Geometry: final body of the model. Coordinates: model frame, mm. Coordinates: 2 decimals unless noted, no trailing zeros. Answer in a Markdown table with one row per item. Add a question column.
1) Ray query, line 1 (X direction, y = 6.5, z = 12.1); line 2 (X direction, y = 5.9, z = 6.5); line 3 (Y direction, x = 6.5, z = 6.9). Return the intervals inside material, ascending. Write a range as from..to.
2) Contact query for flat-ended pins moving along their axis: P1, Ø3.5, axis at x = 7.5, z = 5, coming from the -Y side; P2, Ø5.5, axis at x = 6.5, y = 19.5, coming from the +Z side; P3, Ø5, axis at x = 6.5, z = 6.5, coming from the -Y side. Output: stop coordinate, or through.
3) Section query A-A on z = 8. Count the separate pieces of the cut face and the enclosed holes in it, then the cut area to 3 significant figures.
Solid Edge part; units mm, degrees
sketch "Sketch1" plane through (0, 0, 0) normal (0, 0, 1) x (1, 0, 0)
  line L0 (39, 0) -> (39, 26)
  line L1 (39, 26) -> (0, 26)
  line L2 (0, 26) -> (0, 0)
  line L3 (0, 0) -> (39, 0)
extrude "Protrusion1" add sketch "Sketch1" along normal blind 13
sketch "Sketch2" plane through (6.5, 32.5, 6.5) normal (-1, 0, 0) x (0, -1, 0)
  line L0 (29, 6.5) -> (26, 6.5)
  line L1 (26, 6.5) -> (26, 0)
  line L2 (29, 0) -> (26, 0)
  line L3 (29, 0) -> (29, 1)
  line L4 (29, 1) -> (29.3967, 3.25)
  line L5 (29, 5.5) -> (29.3967, 3.25)
  line L6 (29, 6.5) -> (29, 5.5)
revolve "RevolvedCutout1" cut sketch "Sketch2" angle 360 about axis through (6.5, 6.5, 13) along (0, 0, -1)
chamfer "Chaflán_1" distance 0.75 angle 45 1 edges at (3.5, 6.5, 13)
pattern_linear "Pattern1" count 2 spacing 13 along (0, 1, 0) count 3 spacing 13 along (1, 0, 0) of "RevolvedCutout1", "Chaflán_1"
sketch "Sketch3" plane through (6.5, 32.5, 6.5) normal (-1, 0, 0) x (0, -1, 0)
  line L0 (31.5, 3) -> (32.5, 3)
  line L1 (32.5, 3) -> (32.5, 0)
  line L2 (32.5, 0) -> (31.5, 0)
  line L3 (31.5, 0) -> (26, 0)
  line L4 (26, 0) -> (26, 3)
  line L5 (26, 3) -> (27, 3)
  line L6 (27, 3) -> (29.25, 3.3967)
  line L7 (31.5, 3) -> (29.25, 3.3967)
revolve "RevolvedCutout2" cut sketch "Sketch3" angle 360 about axis through (6.5, 1, 6.5) along (0, 1, 0)
chamfer "Chaflán_2" distance 0.75 angle 45 1 edges at (6.5, 0, 3.5)
pattern_linear "Pattern3" count 3 spacing 13 along (1, 0, 0) of "RevolvedCutout2", "Chaflán_2"
chamfer "Chaflán_531" distance 1.5 angle 45 12 edges at (0, 13, 13) (0, 13, 0) (0, 0, 6.5) (19.5, 0, 13) (19.5, 0, 0) (39, 0, 6.5) (39, 13, 13) (39, 13, 0) (19.5, 26, 13) (19.5, 26, 0) (39, 26, 6.5) (0, 26, 6.5)
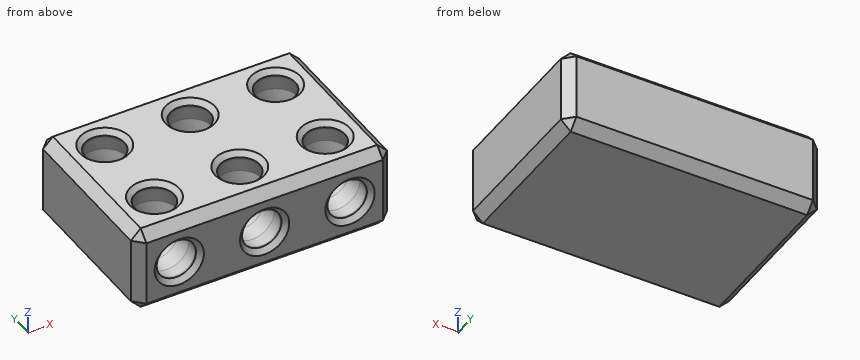
Result:
| question | item | result |
|---|---|---|
| 1 | line 1 | 0.6..3.5, 9.5..16.5, 22.5..29.5, 35.5..38.4 |
| 1 | line 2 | 0..3.5, 9.5..16.5, 22.5..29.5, 35.5..39 |
| 1 | line 3 | 9.5..16.5, 22.5..26 |
| 2 | P1 | y = 0.2 |
| 2 | P2 | z = 6.5 |
| 2 | P3 | y = 6.5 |
| 3 | separate pieces | 1 |
| 3 | enclosed holes | 3 |
| 3 | area | 762 mm2 |
